Can you work these out from the drawing? Everything is in mm from the part's minimum corner. A direction names the side the tool comes from. Coordinates: 2 decimals unless noted, no trailing zeros. Write each loop counter-clockwise with the first axis right and the second up, starting at its lowest first coordinate (ties: lowest second). Pieces come first, ordered by that corner, then holes. Notation, with made-up numbers: (43.5, 71.25) -> (80.5, 71.25) arc R19 cw to (80.5, 106.25) -> close; hole circle Ø5 at (-0.75, 6). An arc over 180 degrees is marked (long way). Use a Markdown table: item, result. Add a question column.
Item 1: Imagine slicing it at C-C, the plane x = 75.5. Write out the boundary of the cut face in (y, z).
Item 2: If I drill on line 1 along X through (y, z) = (6.5, 64); line 2 along Z through (x, y) = (63, 19.5); line 3 along Y through (x, z) = (23, 34.5), over which ranges is the centre line in solid material (lowest first)? Write a range as from..to.
Item 3: If we mould it in two halves opening along Z, with no side actions, what happens to the marked faces 3, 4, 5 and 6? For each: pulls with the +Z half, pulls with the -Z half, needs draft (parallel to the pull), parting line crosses it, or undercut.
Item 4: Imagine slicing it at A-A, the plane x = 37.5. Write out the boundary of the cut face in (y, z), and give its area (3 significant figures).
Item 5: Will this pin go through, and if not, where does the flat tip stop? pin 1 Ø10 at (x, z) = (13.5, 44.5) entering from +Y.
Item 6: Imagine slicing it at D-D, the plane z = 58.5. Write out the boundary of the cut face in (x, y), and give its area (3 significant figures).
Item 7: Imagine slicing it at B-B, the plane y = 6.25. Write out the boundary of the cut face in (x, z), and give its area (3 significant figures).
Item 8: On a 3-axis mill with a long thin cutter (end or side, diameter ignored), from which of +Z, -Z, +X, -X, +Y, -Y can I reach the whole of each face in a straight line? I mean the marked faces 1 and 2. Say none if no direction works.
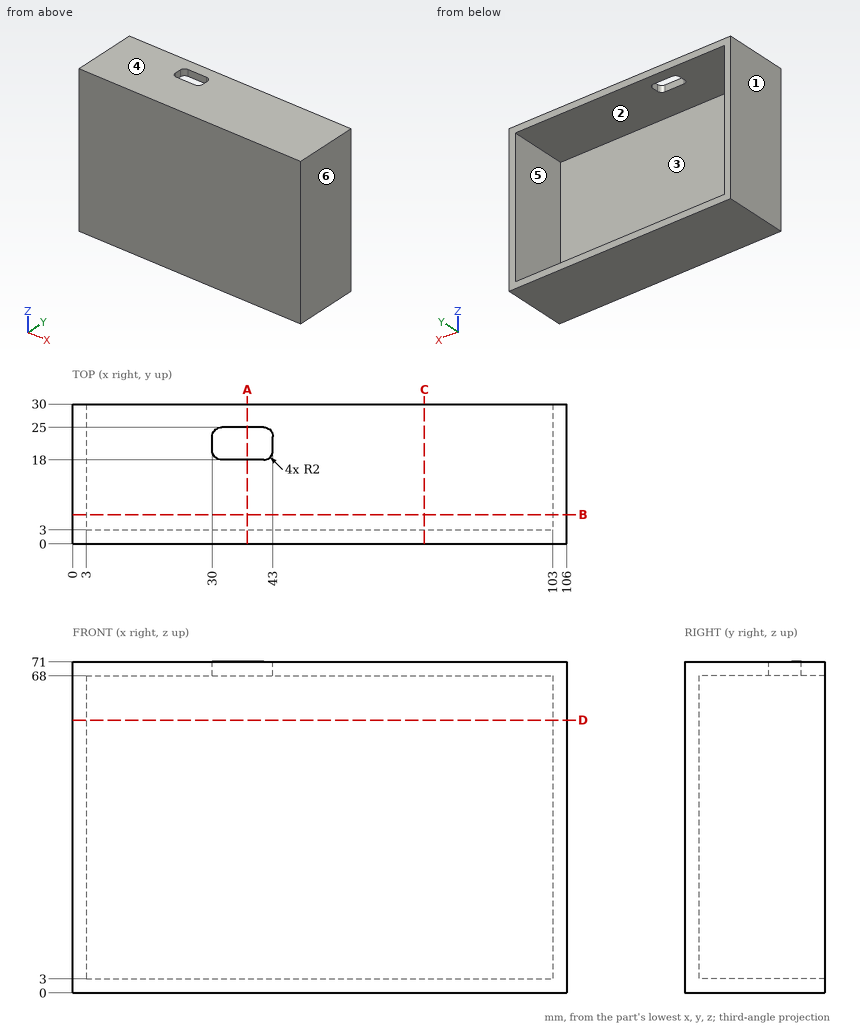
Ans:
| question | item | result |
|---|---|---|
| 1 | outline | (0, 0) -> (30, 0) -> (30, 3) -> (3, 3) -> (3, 68) -> (30, 68) -> (30, 71) -> (0, 71) -> close |
| 2 | line 1 | x = 0..3, 103..106 |
| 2 | line 2 | z = 0..3, 68..71 |
| 2 | line 3 | y = 0..3 |
| 3 | face 3 | undercut |
| 3 | face 4 | pulls with the +Z half |
| 3 | face 5 | undercut |
| 3 | face 6 | needs draft |
| 4 | outline | (0, 0) -> (30, 0) -> (30, 3) -> (3, 3) -> (3, 68) -> (18, 68) -> (18, 71) -> (0, 71) -> close; (25, 68) -> (30, 68) -> (30, 71) -> (25, 71) -> close |
| 4 | area | 354 mm^2 |
| 5 | pin 1 | stops at y = 3 |
| 6 | outline | (0, 0) -> (106, 0) -> (106, 30) -> (103, 30) -> (103, 3) -> (3, 3) -> (3, 30) -> (0, 30) -> close |
| 6 | area | 480 mm^2 |
| 7 | outline | (0, 0) -> (106, 0) -> (106, 71) -> (0, 71) -> close; hole (3, 3) -> (103, 3) -> (103, 68) -> (3, 68) -> close |
| 7 | area | 1,030 mm^2 |
| 8 | face 1 | +Z, -Z, -X, +Y, -Y |
| 8 | face 2 | +Y |
